The model under review builds one solid part; all positions refer to its coordinate system, in mm. A direction names the side the tool comes from. Give positions to 0.01 mm unless a question says otherwise; leave off trailing zeros. Loops run counter-clockwise (first coordinate to the right, second up) from the corner with the lowest first, then second, coordinate; pieces in that order, holes last. Notation, with made-up numbers: (18.25, -3.75) - (42.25, -3.75) arc R16 cw to (42.25, 14.25) - close; hole circle Ø9 at (68, 72.25). An arc over 180 degrees is marked (long way). Return JSON: item names as keys, results as strings. Group by question number.
from build123d import *

# Parameters (mm, degrees)
BOSS_EXTRUDE1_DEPTH     = 6.1
BOSS_EXTRUDE4_START     = -5
BOSS_EXTRUDE4_DEPTH     = 5
BOSS_EXTRUDE5_START     = 5
SKETCH6_R               = 2.75
BOSS_EXTRUDE5_DEPTH     = 5
SKETCH7_R               = 2.75
CUT_EXTRUDE1_DEPTH      = 176.534516689
BOSS_EXTRUDE6_START     = -10
BOSS_EXTRUDE6_DEPTH     = 16.1
CUT_EXTRUDE2_DEPTH      = 192.448730864
CUT_EXTRUDE2_DEPTH_BACK = 192.448730864
SKETCH9_W               = 20.1
SKETCH9_H               = 16.057013855
CUT_EXTRUDE3_DEPTH      = 198.16101231
CUT_EXTRUDE3_DEPTH_BACK = 198.16101231
SKETCH10_R              = 2.75
SKETCH11_R              = 6
CUT_EXTRUDE4_DEPTH      = 192.842324158
SKETCH12_R              = 6
CUT_EXTRUDE5_DEPTH      = 200.499981043
CHAMFER1_SIZE           = 0.25


with BuildPart() as part:
    # Sketch4 → Boss-Extrude1 (new body)
    with BuildSketch(Plane.XY):
        with BuildLine():
            Line((2.791805242, 138.827155544), (104.55323324, 91.375022364))
            Line((104.55323324, 91.375022364), (105.415210237, 92.128353131))
            ThreePointArc((105.415210237, 92.128353131), (9.395226761, 139.684393237), (-92.128353131, 105.415210237))
            Line((-92.128353131, 105.415210237), (-91.375022364, 104.55323324))
            Line((-91.375022364, 104.55323324), (2.791805242, 138.827155544))
        make_face()
    extrude(amount=BOSS_EXTRUDE1_DEPTH)

    # Sketch5 → Boss-Extrude4 (add)
    with BuildSketch(Plane.XY.offset(BOSS_EXTRUDE4_START)):
        with BuildLine():
            Line((30.722164617, 125.803015072), (76.622873865, 104.399162835))
            ThreePointArc((76.622873865, 104.399162835), (87.59255508, 95.382358403), (97.50906947, 85.218726646))
            Line((97.50906947, 85.218726646), (105.415210237, 92.128353131))
            ThreePointArc((105.415210237, 92.128353131), (9.395226761, 139.684393237), (-92.128353131, 105.415210237))
            Line((-92.128353131, 105.415210237), (-85.218726646, 97.50906947))
            ThreePointArc((-85.218726646, 97.50906947), (-30.701883618, 125.807966132), (30.722164617, 125.803015072))
        make_face()
    extrude(amount=BOSS_EXTRUDE4_DEPTH)

    # Sketch6 → Boss-Extrude5 (add)
    with BuildSketch(Plane(origin=(0, 0, -5), x_dir=(-1, 0, 0), z_dir=(0, 0, -1)).offset(BOSS_EXTRUDE5_START)):
        with BuildLine():
            Line((-10, 129.5), (10, 129.5))
            Line((10, 129.5), (10, 109.268365161))
            ThreePointArc((10, 109.268365161), (43.208620922, 100.85926186), (72.205596766, 82.619171024))
            Line((72.205596766, 82.619171024), (92.128353131, 105.415210237))
            ThreePointArc((92.128353131, 105.415210237), (-9.395226761, 139.684393237), (-105.415210237, 92.128353131))
            Line((-105.415210237, 92.128353131), (-82.619171024, 72.205596766))
            ThreePointArc((-82.619171024, 72.205596766), (-49.879754516, 97.732214313), (-10, 109.268365161))
            Line((-10, 109.268365161), (-10, 129.5))
        make_face()
        with Locations((54.966796439, 107.162966034)):
            Circle(SKETCH6_R, mode=Mode.SUBTRACT)
    extrude(amount=-BOSS_EXTRUDE5_DEPTH)

    # Sketch7 → Cut-Extrude1 (cut, through all)
    with BuildSketch(Plane.XY):
        with Locations((76.813119358, 91.542310953)):
            Circle(SKETCH7_R)
    extrude(amount=-CUT_EXTRUDE1_DEPTH, mode=Mode.SUBTRACT)

    # Sketch8 → Boss-Extrude6 (add)
    with BuildSketch(Plane.XY.offset(BOSS_EXTRUDE6_START)):
        with BuildLine():
            Line((-10.05, 139.638810866), (-10.05, 159.5))
            Line((-10.05, 159.5), (-75.100690367, 118.15196277))
            ThreePointArc((-75.100690367, 118.15196277), (-43.909921177, 132.935769536), (-10.05, 139.638810866))
        make_face()
        with BuildLine():
            Line((10.05, 139.638810866), (10.05, 159.5))
            Line((10.05, 159.5), (75.100690367, 118.15196277))
            ThreePointArc((75.100690367, 118.15196277), (43.909921177, 132.935769536), (10.05, 139.638810866))
        make_face()
    extrude(amount=BOSS_EXTRUDE6_DEPTH)

    # Sketch9 → Cut-Extrude2 (cut, two sides: drawn at the far end of the back side and taken through both)
    with BuildSketch(Plane.XY.offset(-CUT_EXTRUDE2_DEPTH_BACK)):
        with Locations((0, 147.528506928)):
            Rectangle(SKETCH9_W, SKETCH9_H)
    extrude(amount=CUT_EXTRUDE2_DEPTH + CUT_EXTRUDE2_DEPTH_BACK, mode=Mode.SUBTRACT)

    # Sketch10 → Cut-Extrude3 (cut, two sides: drawn at the far end of the back side and taken through both)
    with BuildSketch(Plane(origin=(-10.05, 0, 0), x_dir=(0, 0, -1), z_dir=(1, 0, 0)).offset(-CUT_EXTRUDE3_DEPTH_BACK)):
        with Locations(Location((1.95, 149.5, 0), (0, 0, 90))):
            Circle(SKETCH10_R)
    extrude(amount=CUT_EXTRUDE3_DEPTH + CUT_EXTRUDE3_DEPTH_BACK, mode=Mode.SUBTRACT)

    # Sketch11 → Cut-Extrude4 (cut, through all)
    with BuildSketch(Plane(origin=(14, 0, 0), x_dir=(0, 0, -1), z_dir=(1, 0, 0))):
        with Locations(Location((1.95, 149.5, 0), (0, 0, 90))):
            Circle(SKETCH11_R)
    extrude(amount=CUT_EXTRUDE4_DEPTH, mode=Mode.SUBTRACT)

    # Sketch12 → Cut-Extrude5 (cut, through all)
    with BuildSketch(Plane(origin=(-14, 0, 0), x_dir=(0, 0, -1), z_dir=(1, 0, 0))):
        with Locations(Location((1.95, 149.5, 0), (0, 0, 90))):
            Circle(SKETCH12_R)
    extrude(amount=-CUT_EXTRUDE5_DEPTH, mode=Mode.SUBTRACT)

    # Chamfer1
    chamfer1_edges = [part.edges().sort_by_distance(p)[0] for p in [
        (0, 139.5, -10),
        (10, 119.384182581, -10),
        (0, 129.5, -10),
        (-10, 119.384182581, -10),
        (10.05, 149.5, -10),
        (-10.05, 149.5, -10),
    ]]
    chamfer(chamfer1_edges, length=CHAMFER1_SIZE)


solid = part.part
Item 1: Take a section at D-D (x = 50). State the section outline as (y, z) points.
Item 2: Take a section at C-C (y = 149.5). State the section outline as (x, z) points, then the cut area to 3 significant figures.
Item 3: Take a section at B-B (z = -1.95). State the section outline as (x, y) points.
Item 4: Take a section at A-A (y = 101.5). State the section outline as (x, z) points.
Item 5: For P1, Ø5, axis at y = 122, z = -6, coming from the -X side; P2, Ø3, axis at x = 39, y = 110, coming from the +Z side; P3, Ø5, axis at y = 147, z = -3.5, coming from the -X side; P4, Ø15.5, axis at x = 91, y = 94, coming from the +Z side, all flat-tipped, find the tip position at first contact; note any pin that passes through.
Item 6: For L1, parallel to Z at x = -14, y = 127; L2, parallel to Y at x = 11.8, z = -1.95; L3, parallel to X at y = 110, z = -6.25, list the stretches that pass through material, from the lowest coordinate up. Write a range as from..to.
Item 7: Tool access review of faces 1 (the face through (-10.05, 147, 0)), 2 (the face through (0, 129.5, -7)), 3 (the face through (79.353, 90.489, -7.465)), 4 (the face through (54, 103, -5)), 5 (the face through (-22.254, 143.506, -1.686)): name each direction out of +Z, -Z, +X, -X, +Y, -Y from which nothing blocks a thin tool from reaching the whole face with its end or side.
Item 8: Mouldability with a two-part tool opening along Y and no side actions: class faces 6 (the face through (10.05, 147, -4)), 7 (the face through (-12.05, 152.12, -1.12)), 8 (the face through (90.98, 106.41, -2.06)) as +Y half, -Y half, draft (parallel to the pull), parting line (faces both ways), or undercut.
Check sheet entries:
{
 "1": {"outline": "(97.67, -10) - (134.11, -10) - (134.11, 6.1) - (116.81, 6.1) - (116.81, -5) - (97.67, -5) - close"},
 "2": {"outline": "(-25.78, -10) - (-10.3, -10) - (-10.05, -9.75) - (-10.05, -4.7) - (-14, -4.7) - (-14, -7.95) - (-25.78, -7.95) - close; (-25.78, 4.05) - (-14, 4.05) - (-14, 0.8) - (-10.05, 0.8) - (-10.05, 6.1) - (-25.78, 6.1) - close; (10.05, -9.75) - (10.3, -10) - (25.78, -10) - (25.78, -7.95) - (14, -7.95) - (14, -4.7) - (10.05, -4.7) - close; (10.05, 0.8) - (14, 0.8) - (14, 4.05) - (25.78, 4.05) - (25.78, 6.1) - (10.05, 6.1) - close", "area": "180 mm^2"},
 "3": {"outline": "(-92.13, 105.42) - (-85.22, 97.51) arc R129.5 cw to (30.72, 125.8) - (76.62, 104.4) arc R129.5 cw to (97.51, 85.22) - (105.42, 92.13) arc R140 ccw to (75.1, 118.15) - (35.22, 143.5) - (14, 143.5) - (14, 146.75) - (10.05, 146.75) - (10.05, 139.5) - (-10.05, 139.5) - (-10.05, 146.75) - (-14, 146.75) - (-14, 143.5) - (-35.22, 143.5) - (-75.1, 118.15) arc R140 ccw to start; (-16.34, 155.5) - (-14, 155.5) - (-14, 152.25) - (-10.05, 152.25) - (-10.05, 159.5) - close; (10.05, 152.25) - (14, 152.25) - (14, 155.5) - (16.34, 155.5) - (10.05, 159.5) - close"},
 "4": {"outline": "(-88.71, -10) - (-41.68, -10) - (-41.68, -5) - (-80.42, -5) - (-80.42, 0) - (-88.71, 0) - close; (41.68, -10) - (96.42, -10) - (96.42, 6.1) - (82.84, 6.1) - (82.84, 0) - (80.42, 0) - (80.42, -5) - (41.68, -5) - close"},
 "5": {"P1": "stops at x = -72.98", "P2": "stops at z = -5", "P3": "stops at x = -14", "P4": "stops at z = 6.1"},
 "6": {"L1": "z = -10..-5", "L2": "y = 128.96..146.75, 152.25..158.39", "L3": "x = -86.6..-10, 10..86.6"},
 "7": {"face 1": "+Z, -Z, +Y", "face 2": "-Z, -Y", "face 3": "+Z, -Z", "face 4": "+Z, -Y", "face 5": "-X"},
 "8": {"face 6": "draft", "face 7": "undercut", "face 8": "+Y half"}
}
